Input: dimensioned drawing with shaded views. Units: mm. Origin: part minimum x, y, z. Round coordinates to 2 decimals unless told otherwise and drop trailing zeros. Order: outer loops, then holes, each group sorted by start corner. A loop starts at its lowest first (then second) coordinate and runs counter-clockwise, first axis right, second up. Notation, with made-up numbers: M 49.25,46 L 93.25,46 A14 ccw 93.25,52 Z; hole C -29.75,76.5 d4. An arc over 180 degrees is marked long. Put each result on its own line as item: value. Start each with the question number.
1) First-contact query: P1, Ø4, axis at x = 12, z = 19, coming from the +Y side; P2, Ø1, axis at x = 4, z = 17, coming from the +Y side. Flat tips, straight axial feed; report the tip coordinate or a pass-through.
2) Section A-A, the plane z = 22.5. Return loops of the section in (x, y), then the cut area to 3 significant figures.
3) Section B-B, the plane x = 4. Return loops of the section in (y, z), then the cut area to 3 significant figures.
4) Section C-C, the plane x = 1.5. Return loops of the section in (y, z), then the cut area to 3 significant figures.
5) Material intervals for probe 1 along Y at (x, z) = (9.75, 8.5); probe 2 along Y at (x, z) = (8.75, 10); probe 3 along X at (y, z) = (50.5, 6.5), sorted ascending. Write a range as [from, to].
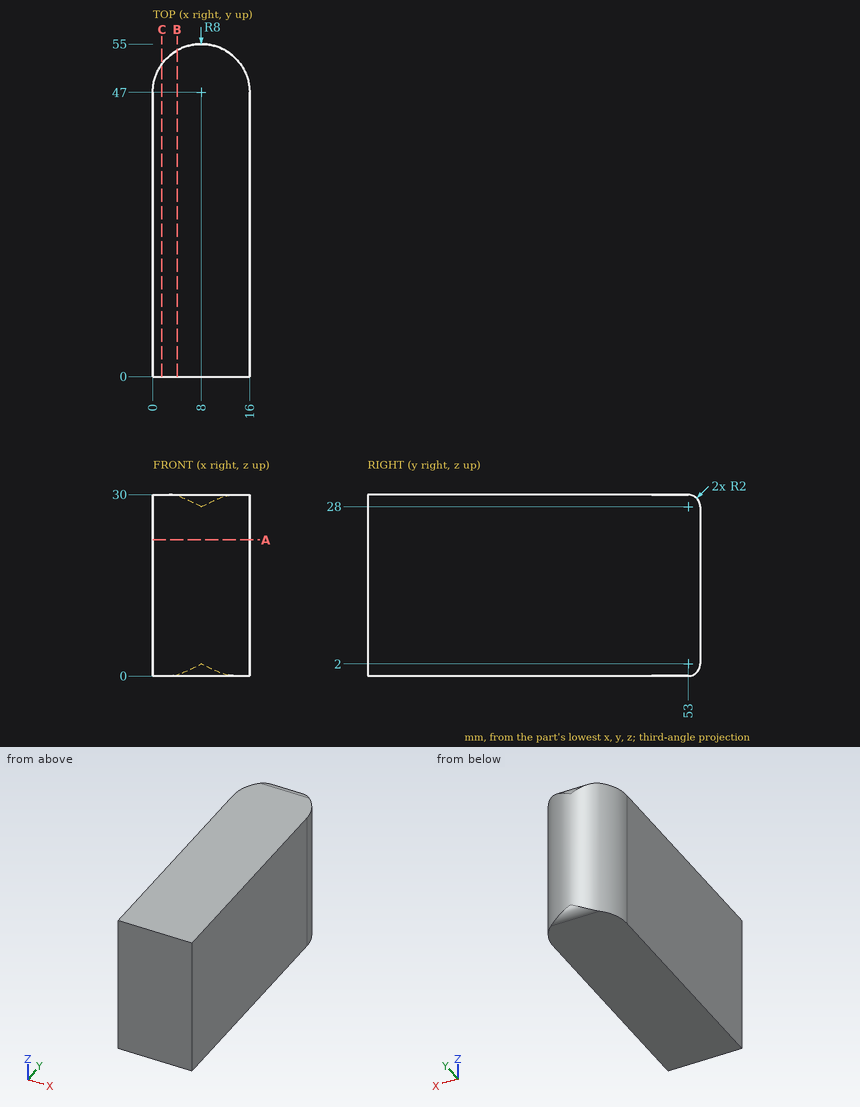
Result sheet:
1. P1: stops at y = 54.75
1. P2: stops at y = 54.19
2. outline: M 0,0 L 16,0 L 16,47 A8 ccw 0,47 Z
2. area: 853 mm2
3. outline: M 0,0 L 53,0 A2 ccw 53.93,0.23 L 53.93,29.77 A2 ccw 53,30 L 0,30 Z
3. area: 1,620 mm2
4. outline: M 0,0 L 51.66,0 L 51.66,30 L 0,30 Z
4. area: 1,550 mm2
5. probe 1: y = [0, 54.81]
5. probe 2: y = [0, 54.96]
5. probe 3: x = [0.81, 15.19]
